Design review of the part built by this model. Coordinates are the model's own, in mm. Give positions to 0.01 mm unless a question says otherwise; leave off trailing zeros. Order: outer loops, then holes, each group sorted by start corner. A loop starts at its lowest first (then second) coordinate and runs counter-clockwise, first axis right, second up. Notation, with made-up numbers: (76.25, 74.25) - (117.25, 74.25) arc R25 cw to (117.25, 91.25) - close; hole circle Ø1 at (-30, -3.75). An arc over 180 degrees is marked (long way). Write each question's results on one line, items separated by ' | '. Start each with the question number.
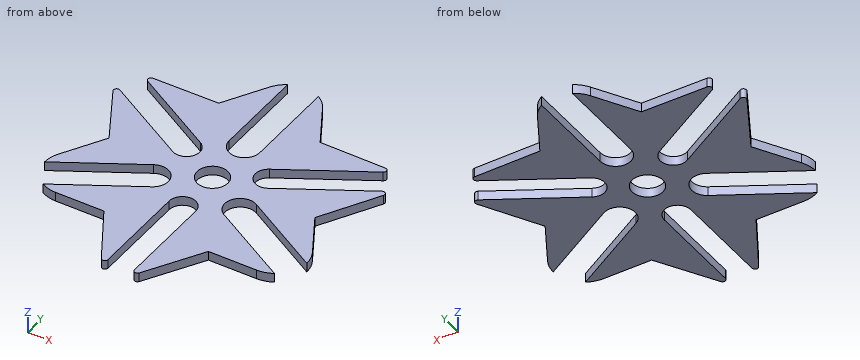
```python
from build123d import *

# Parameters (mm, degrees)
SKETCH1_R           = 5
BOSS_EXTRUDE1_DEPTH = 3
FILLET1_R           = 1


with BuildPart() as part:
    # Sketch1 → Boss-Extrude1 (new body)
    with BuildSketch(Plane.XY):
        with BuildLine():
            Line((-5, 46.395280957), (-5, 16.395280957))
            ThreePointArc((-5, 16.395280957), (0, 11.395280957), (5, 16.395280957))
            Line((5, 16.395280957), (5, 46.395280957))
            ThreePointArc((5, 46.395280957), (7.071067812, 44.806094731), (8.660254038, 42.735026919))
            Line((8.660254038, 42.735026919), (16.5, 29.156188594))
            Line((16.5, 29.156188594), (41.509870079, 28.940674337))
            Line((41.509870079, 28.940674337), (11.198980946, 11.440674337))
            ThreePointArc((11.198980946, 11.440674337), (9.621988261, 5.555257513), (15.507405085, 3.978264828))
            Line((15.507405085, 3.978264828), (45.818294218, 21.478264828))
            Line((45.818294218, 21.478264828), (33.5, -0.288675135))
            Line((33.5, -0.288675135), (41.339745962, -13.867513459))
            ThreePointArc((41.339745962, -13.867513459), (42.338750187, -16.279323008), (42.679491924, -18.867513459))
            Line((42.679491924, -18.867513459), (16.698729811, -3.867513459))
            ThreePointArc((16.698729811, -3.867513459), (9.868602792, -5.697640478), (11.698729811, -12.527767497))
            Line((11.698729811, -12.527767497), (37.679491924, -27.527767497))
            ThreePointArc((37.679491924, -27.527767497), (35.267682375, -28.526771722), (32.679491924, -28.867513459))
            Line((32.679491924, -28.867513459), (17, -28.867513459))
            Line((17, -28.867513459), (4.308424139, -50.418939165))
            Line((4.308424139, -50.418939165), (4.308424139, -15.418939165))
            ThreePointArc((4.308424139, -15.418939165), (0, -11.110515025), (-4.308424139, -15.418939165))
            Line((-4.308424139, -15.418939165), (-4.308424139, -50.418939165))
            Line((-4.308424139, -50.418939165), (-17, -28.867513459))
            Line((-17, -28.867513459), (-32.679491924, -28.867513459))
            ThreePointArc((-32.679491924, -28.867513459), (-35.267682375, -28.526771722), (-37.679491924, -27.527767497))
            Line((-37.679491924, -27.527767497), (-11.698729811, -12.527767497))
            ThreePointArc((-11.698729811, -12.527767497), (-9.868602792, -5.697640478), (-16.698729811, -3.867513459))
            Line((-16.698729811, -3.867513459), (-42.679491924, -18.867513459))
            ThreePointArc((-42.679491924, -18.867513459), (-42.338750187, -16.279323008), (-41.339745962, -13.867513459))
            Line((-41.339745962, -13.867513459), (-33.5, -0.288675135))
            Line((-33.5, -0.288675135), (-45.818294218, 21.478264828))
            Line((-45.818294218, 21.478264828), (-15.507405085, 3.978264828))
            ThreePointArc((-15.507405085, 3.978264828), (-9.621988261, 5.555257513), (-11.198980946, 11.440674337))
            Line((-11.198980946, 11.440674337), (-41.509870079, 28.940674337))
            Line((-41.509870079, 28.940674337), (-16.5, 29.156188594))
            Line((-16.5, 29.156188594), (-8.660254038, 42.735026919))
            ThreePointArc((-8.660254038, 42.735026919), (-7.071067812, 44.806094731), (-5, 46.395280957))
        make_face()
        Circle(SKETCH1_R, mode=Mode.SUBTRACT)
    extrude(amount=BOSS_EXTRUDE1_DEPTH)

    # Fillet1
    fillet1_edges = [part.edges().sort_by_distance(p)[0] for p in [
        (41.509870079, 28.940674337, 1.5),
        (45.818294218, 21.478264828, 1.5),
        (4.308424139, -50.418939165, 1.5),
        (-4.308424139, -50.418939165, 1.5),
        (-45.818294218, 21.478264828, 1.5),
        (-41.509870079, 28.940674337, 1.5),
    ]]
    fillet(fillet1_edges, radius=FILLET1_R)


solid = part.part
```
Q1. For line 1 (Y direction, x = 0, z = 1.75); line 2 (Y direction, x = 36, z = 1.85); line 3 (Y direction, x = 29.5, z = 0.3), list the stretches that pass through material, from the lowest coordinate up. Write a range as [from, to].
Q2. Add section B-B (x = -24.5). Give the boundary of the cut face in (y, z), plus the area to 3 significant figures.
Q3. Add section A-A (x = 0). Give the boundary of the cut face in (y, z), plus the area to 3 significant figures.
Q4. Insertion check: pin 1 Ø1.5 at (x, z) = (-31, 2) entering from +Y; pin 2 Ø1.5 at (y, z) = (37.5, 1) entering from +X; pin 3 Ø0.9 at (y, z) = (-23.5, 1) entering from -X. Each pin has a flat end and moves straight along its axis. Give the tip position at first contact, or say it passes through.
Verdict:
1) line 1: y = [-11.11, -5], [5, 11.4] | line 2: y = [-28.3, -26.56], [-15.01, -4.62], [4.13, 15.81], [25.76, 28.99] | line 3: y = [-28.87, -22.81], [-11.26, 12.06], [22.01, 29.04]
2) outline: (-28.87, 0) - (-19.92, 0) - (-19.92, 3) - (-28.87, 3) - close; (-8.37, 0) - (9.17, 0) - (9.17, 3) - (-8.37, 3) - close; (19.12, 0) - (29.09, 0) - (29.09, 3) - (19.12, 3) - close | area: 109 mm2
3) outline: (-11.11, 0) - (-5, 0) - (-5, 3) - (-11.11, 3) - close; (5, 0) - (11.4, 0) - (11.4, 3) - (5, 3) - close | area: 37.5 mm2
4) pin 1: stops at y = 29.04 | pin 2: stops at x = 12.12 | pin 3: stops at x = -31.48
